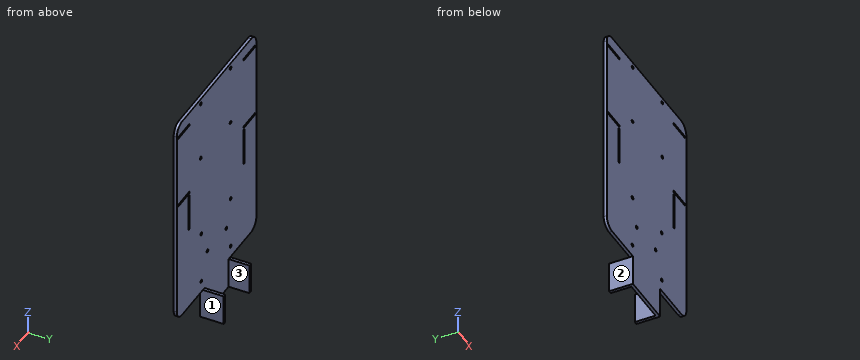
```python
from build123d import *

# Parameters (mm, degrees)
BOSS_EXTRUDE1_DEPTH     = 3
SKETCH2_R               = 1.6
SKETCH2_W               = 21.700006253
SKETCH2_H               = 2
SKETCH2_W_2             = 2
SKETCH2_H_2             = 37.126830638
CUT_EXTRUDE1_DEPTH      = 155.463587942
SKETCH3_W               = 3
SKETCH3_H               = 30
BOSS_EXTRUDE2_DEPTH     = 20
FILLET2_R               = 10
CUT_EXTRUDE2_DEPTH      = 157.137759687
CUT_EXTRUDE2_DEPTH_BACK = 157.137759687
SKETCH5_R               = 1.6


with BuildPart() as part:
    # Sketch1 → Boss-Extrude1 (new body)
    with BuildSketch(Plane(origin=(0, 0, 0), x_dir=(1, 0, 0), z_dir=(0, 1, 0))):
        Polygon((-75, 105), (-25.75, 105), (-25.75, 135), (25.75, 135), (25.75, 105), (75, 105), (75, -105), (-75, -105), align=None)
    extrude(amount=BOSS_EXTRUDE1_DEPTH)

    # Sketch2 → Cut-Extrude1 (cut, through all)
    with BuildSketch(Plane(origin=(0, 3, 0), x_dir=(1, 0, 0), z_dir=(0, 1, 0))):
        with Locations(Location((-26.500321166, 93.505677214, 0), (0, 0, 270))):
            Circle(SKETCH2_R)
        with Locations(Location((28.569678834, 93.505677214, 0), (0, 0, 270))):
            Circle(SKETCH2_R)
        with Locations(Location((28.569678834, 42.065677214, 0), (0, 0, 270))):
            Circle(SKETCH2_R)
        with Locations(Location((-26.500321166, 42.065677214, 0), (0, 0, 270))):
            Circle(SKETCH2_R)
        with Locations(Location((-26.398287195, -40.891541183, 0), (0, 0, 270))):
            Circle(SKETCH2_R)
        with Locations(Location((29.601712805, -40.891541183, 0), (0, 0, 270))):
            Circle(SKETCH2_R)
        with Locations(Location((-26.398287195, -99.891541183, 0), (0, 0, 270))):
            Circle(SKETCH2_R)
        with Locations(Location((29.601712805, -99.891541183, 0), (0, 0, 270))):
            Circle(SKETCH2_R)
        with Locations((61.56254881, -18.52352323)):
            Rectangle(SKETCH2_W, SKETCH2_H)
        with Locations((-61.56254881, -18.52352323)):
            Rectangle(SKETCH2_W, SKETCH2_H)
        with Locations((51.712545683, 2.74325537)):
            Rectangle(SKETCH2_W_2, SKETCH2_H_2)
        with Locations((-51.712545683, 2.74325537)):
            Rectangle(SKETCH2_W_2, SKETCH2_H_2)
        with Locations((61.56254881, -91.993921103)):
            Rectangle(SKETCH2_W, SKETCH2_H)
        with Locations((-61.56254881, -91.993921103)):
            Rectangle(SKETCH2_W, SKETCH2_H)
    extrude(amount=-CUT_EXTRUDE1_DEPTH, mode=Mode.SUBTRACT)

    # Sketch3 → Boss-Extrude2 (add)
    with BuildSketch(Plane(origin=(0, 3, 0), x_dir=(1, 0, 0), z_dir=(0, 1, 0))):
        with Locations((-24.25, 120)):
            Rectangle(SKETCH3_W, SKETCH3_H)
        with Locations((24.25, 120)):
            Rectangle(SKETCH3_W, SKETCH3_H)
    extrude(amount=BOSS_EXTRUDE2_DEPTH)

    # Fillet2
    fillet2_edges = [part.edges().sort_by_distance(p)[0] for p in [
        (75, 1.5, 105),
        (-75, 1.5, 105),
        (-75, 1.5, -105),
        (75, 1.5, -105),
    ]]
    fillet(fillet2_edges, radius=FILLET2_R)

    # Sketch5 → Cut-Extrude2 (cut, two sides: drawn at the far end of the back side and taken through both)
    with BuildSketch(Plane.XZ.offset(-CUT_EXTRUDE2_DEPTH_BACK)):
        with Locations(Location((-18.452668306, -68.632073291, 0), (0, 0, 90))):
            Circle(SKETCH5_R)
        with Locations(Location((17.047331694, -68.632073291, 0), (0, 0, 90))):
            Circle(SKETCH5_R)
    extrude(amount=CUT_EXTRUDE2_DEPTH + CUT_EXTRUDE2_DEPTH_BACK, mode=Mode.SUBTRACT)


solid = part.part
```
The model under review builds one solid part; all positions refer to its coordinate system, in mm. Face numbers are marked on the shaded views. Round coordinates to 2 decimals unless told otherwise and drop trailing zeros. Write each loop counter-clockwise with the first axis right and the second up, starting at its lowest first coordinate (ties: lowest second). Pieces come first, ordered by that corner, then holes. Notation, with made-up numbers: (8.25, 29) - (67.25, 29) arc R31 ccw to (67.25, 62) - close; hole circle Ø10 at (15, 45.25). An arc over 180 degrees is marked (long way). One line per question, with ' | ' between items.
Item 1: Add section B-B, the plane z = 4. Give the boundary of the cut face in (x, y).
Resolved:
outline: (-75, 0) - (-52.71, 0) - (-52.71, 3) - (-75, 3) - close; (-50.71, 0) - (50.71, 0) - (50.71, 3) - (-50.71, 3) - close; (52.71, 0) - (75, 0) - (75, 3) - (52.71, 3) - close
Item 2: For P1, Ø10, axis at y = 12, z = -121.5, coming from the -X side; P2, Ø0.9, axis at x = 64.5, y = 1.5, coming from the -Z side; P3, Ø4, axis at x = -16.5, z = -90.5, coming from the +Y side; P4, Ø4, axis at x = 29.6, z = 40.89, coming from the -Y side, all flat-tipped, find the tip position at first contact; note any pin that passes through.
Resolved:
P1: stops at x = -25.75 | P2: stops at z = -105 | P3: stops at y = 3 | P4: stops at y = 0
Item 3: To check wall thickness, follow probe 1 along X at (y, z) = (12.5, -112); probe 2 along Y at (x, z) = (16.5, 22); probe 3 along Z at (x, y) = (-24.5, 18.75). State the ranges of each line that lie inside material, in increasing order.
Resolved:
probe 1: x = -25.75 to -22.75, 22.75 to 25.75 | probe 2: y = 0 to 3 | probe 3: z = -135 to -105
Item 4: Add section C-C, the plane x = 6. Give the boundary of the cut face in (y, z), then the cut area to 3 significant figures.
Resolved:
outline: (0, -135) - (3, -135) - (3, 105) - (0, 105) - close | area: 720 mm2
Item 5: Add section D-D, the plane z = 84. Give the boundary of the cut face in (x, y), then the cut area to 3 significant figures.
Resolved:
outline: (-75, 0) - (75, 0) - (75, 3) - (-75, 3) - close | area: 450 mm2
Item 6: The part is to be moulded in two halves that separate along X. For the marked faces 1, 2 and 3, say which applies: pulls with the +X half, pulls with the -X half, needs draft (parallel to the pull), parting line crosses it, or undercut.
Resolved:
face 1: pulls with the +X half | face 2: pulls with the -X half | face 3: undercut
Item 7: Add section A-A, the plane y = 20.5. Give the boundary of the cut face in (x, z).
Resolved:
outline: (-25.75, -135) - (-22.75, -135) - (-22.75, -105) - (-25.75, -105) - close; (22.75, -135) - (25.75, -135) - (25.75, -105) - (22.75, -105) - close
